Can you work these out from the model? Positions are in its coordinate system, mm. A direction names the side the tool comes from. Round coordinates to 2 decimals unless told otherwise and drop trailing zeros. Write each loop counter-clockwise with the first axis right and the second up, starting at its lowest first coordinate (ties: lowest second). Pieces come first, ordered by that corner, then holes.
Q1. If we section it at A-A (y = 5.75): Please give me the cut outline in (x, z) (3 decimals).
Q2. For faces 1 (the flat face through (16, 0, 229)), 2 (the flat face through (28.575, 8, 229)), which set-ups out of +Z, -Z, +X, -X, +Y, -Y let a thin tool reach every point of the face, with its end or its side?
Q3. If we section it at B-B (z = 109): Please give me the cut outline in (x, y) (3 decimals).
Q4. I'm going to push flat-ended pins straight in: pin 1 Ø12.5 at (x, z) = (20, 343.5) entering from +Y (3 decimals); pin 2 Ø4.5 at (x, z) = (15.88, 458.79) entering from -Y. Where does each tip first touch, or does it pass through?
Q5. If we section it at C-C (x = 23): Please give me the cut outline in (y, z) (3 decimals).
Q6. Please list where these lines run through material, in increasing order: line 1 along X through (y, z) = (9.75, 325) (3 decimals); line 2 along Y through (x, z) = (24.5, 362.5) (3 decimals).
Q7. We'd pull the mould along X, two halves only. Please class faces 3 (the flat face through (0, 6, 229)), 4 (the flat face through (16, 3.175, 229)), 5 (the flat face through (16, 2, 0)): +X half, -X half, draft (parallel to the pull), parting line (faces both ways), or undercut.
from build123d import *

# Parameters (mm, degrees)
BOSS_EXTRUDE1_DEPTH = 463.55
CUT_EXTRUDE1_REACH  = 466.734
SKETCH2_R           = 2.413
CUT_EXTRUDE2_REACH  = 466.734
SKETCH3_R           = 2.413


with BuildPart() as part:
    # Sketch1 → Boss-Extrude1 (new body)
    with BuildSketch(Plane.XY):
        Polygon((3.175, 3.175), (3.175, 12.7), (0, 12.7), (0, 0), (31.75, 0), (31.75, 12.7), (28.575, 12.7), (28.575, 3.175), align=None)
    extrude(amount=BOSS_EXTRUDE1_DEPTH)

    # Sketch2 → Cut-Extrude1 (cut, up to next)
    with BuildSketch(Plane(origin=(0, 3.175, 0), x_dir=(1, 0, 0), z_dir=(0, 1, 0)), mode=Mode.PRIVATE) as cut_extrude1_sk1:
        with Locations(Location((15.875, -458.7875, 0), (0, 0, 270))):
            Circle(SKETCH2_R)
    cut_extrude1_tool1 = extrude(cut_extrude1_sk1.sketch, amount=-CUT_EXTRUDE1_REACH, mode=Mode.PRIVATE) & part.part
    # Sketch2 → Cut-Extrude1 (cut, up to next)
    with BuildSketch(Plane(origin=(0, 3.175, 0), x_dir=(1, 0, 0), z_dir=(0, 1, 0)), mode=Mode.PRIVATE) as cut_extrude1_sk2:
        with Locations(Location((15.875, -4.7625, 0), (0, 0, 270))):
            Circle(SKETCH2_R)
    cut_extrude1_tool2 = extrude(cut_extrude1_sk2.sketch, amount=-CUT_EXTRUDE1_REACH, mode=Mode.PRIVATE) & part.part
    add(cut_extrude1_tool1.solids().sort_by_distance((15.875, 3.175, 458.7875))[0], mode=Mode.SUBTRACT)
    add(cut_extrude1_tool2.solids().sort_by_distance((15.875, 3.175, 4.7625))[0], mode=Mode.SUBTRACT)

    # Sketch3 → Cut-Extrude2 (cut, up to next)
    with BuildSketch(Plane(origin=(0, 3.175, 0), x_dir=(1, 0, 0), z_dir=(0, 1, 0)), mode=Mode.PRIVATE) as cut_extrude2_sk1:
        with Locations(Location((15.875, -231.775, 0), (0, 0, 270))):
            Circle(SKETCH3_R)
    cut_extrude2_tool1 = extrude(cut_extrude2_sk1.sketch, amount=-CUT_EXTRUDE2_REACH, mode=Mode.PRIVATE) & part.part
    add(cut_extrude2_tool1.solids().sort_by_distance((15.875, 3.175, 231.775))[0], mode=Mode.SUBTRACT)


solid = part.part
A:
1. outline: (0, 0) - (3.175, 0) - (3.175, 463.55) - (0, 463.55) - close; (28.575, 0) - (31.75, 0) - (31.75, 463.55) - (28.575, 463.55) - close
2. face 1: +Z, -Z, +X, -X, -Y
2. face 2: +Z, -Z, +Y
3. outline: (0, 0) - (31.75, 0) - (31.75, 12.7) - (28.575, 12.7) - (28.575, 3.175) - (3.175, 3.175) - (3.175, 12.7) - (0, 12.7) - close
4. pin 1: stops at y = 3.175
4. pin 2: passes through
5. outline: (0, 0) - (3.175, 0) - (3.175, 463.55) - (0, 463.55) - close
6. line 1: x = 0 to 3.175, 28.575 to 31.75
6. line 2: y = 0 to 3.175
7. face 3: -X half
7. face 4: undercut
7. face 5: draft
